Design review of the part shown in the three views and the two pictorial views. Dimensions are in mm from the part's minimum x, y and z. Give positions to 0.01 mm unless a question says otherwise; leave off trailing zeros. Order: outer loops, then holes, each group sorted by start corner. A loop starts at its lowest first (then second) coordinate and runs counter-clockwise, first axis right, second up. Notation, with made-up numbers: M 15.25,39 L 73.25,39 A19 cw 73.25,44 Z; hole C -22,27 d8. An arc over 180 degrees is marked long. Answer as a JSON object with one key per item and string values.
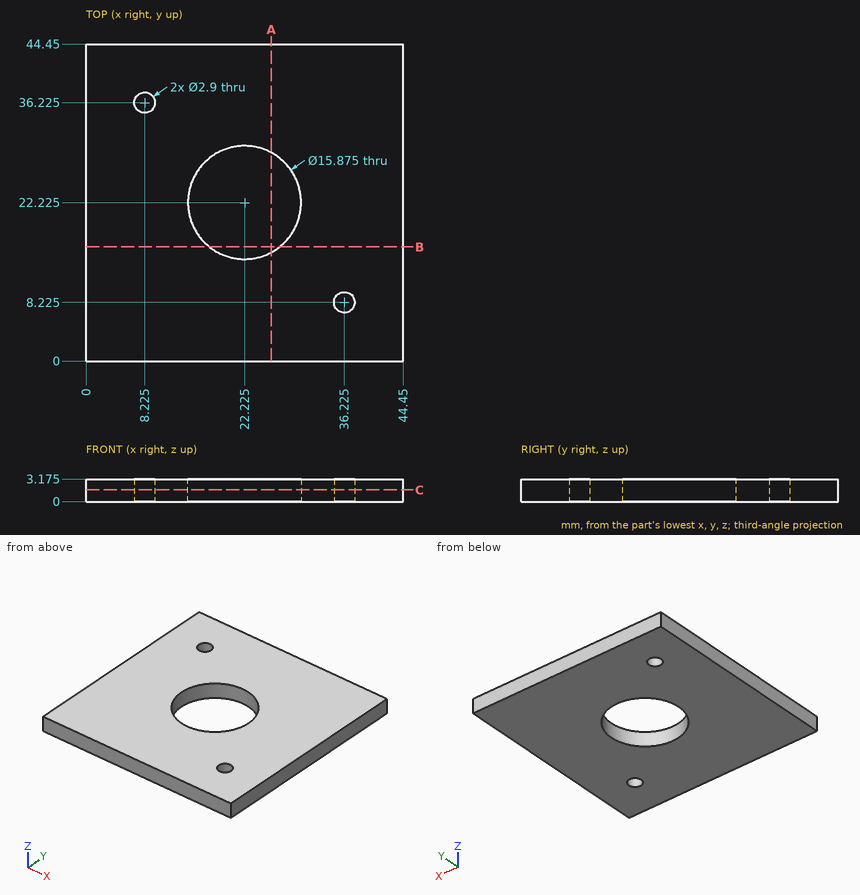
(1) We need section B-B (y = 16). Write out the cut boundary in (x, z) (3 decimals).
Checked values:
{"outline": "M 0,0 L 17.3,0 L 17.3,3.175 L 0,3.175 Z; M 27.15,0 L 44.45,0 L 44.45,3.175 L 27.15,3.175 Z"}
(2) We need section A-A (x = 26). Write out the cut boundary in (y, z) (3 decimals), plus the area to 3 significant figures.
Checked values:
{"outline": "M 0,0 L 15.243,0 L 15.243,3.175 L 0,3.175 Z; M 29.207,0 L 44.45,0 L 44.45,3.175 L 29.207,3.175 Z", "area": "96.8 mm^2"}
(3) Insertion check: pin 1 (10 mm diameter, centred on x = 17.5, y = 26, fed in from +Z) (3 decimals); pin 2 (2.5 mm diameter, centred on x = 36.225, y = 8.225, fed in from -Z). Each pin has a flat end and moves straight along its axis. Give the tip position at first contact, or say it passes through.
Checked values:
{"pin 1": "stops at z = 3.175", "pin 2": "passes through"}
(4) We need section C-C (z = 1.65). Count the separate pieces of the cut face and the enclosed holes in it, plus the area to 3 significant figures.
Checked values:
{"separate pieces": "1", "enclosed holes": "3", "area": "1,760 mm^2"}
(5) To check wall thickness, follow L1, parallel to Y at x = 22.5, z = 2.8; L2, parallel to X at y = 21, z = 2.15; L3, parallel to X at y = 18, z = 2.5. State the ranges of each line that lie inside material, in increasing order. Write a range as from..to.
Checked values:
{"L1": "y = 0..14.29, 30.16..44.45", "L2": "x = 0..14.38, 30.07..44.45", "L3": "x = 0..15.51, 28.94..44.45"}
